Can you work these out from the model? Positions are in its coordinate system, mm. A direction names the side the tool comes from. Round coordinates to 2 decimals unless told otherwise and drop trailing zeros. Write each loop counter-clockwise with the first axis right and the second up, starting at its lowest first coordinate (ties: lowest second). Pieces come first, ordered by that corner, then holes. Notation, with made-up numbers: (13.25, -1) -> (61.25, -1) arc R26 cw to (61.25, 37) -> close; hole circle Ø11 at (27.25, 65). An arc over 180 degrees is marked (long way). Write item = value, one per line. Start each with the question number.
1) Imagine slicing it at B-B, the plane z = 10. Please give me the cut outline in (x, y).
2) Thinking about a two-plate mould opening in X: for faces 6 (the face through (-27, 17, 15)), 7 (the face through (0, 13, 17)), 8 (the face through (24.465, 23.171, 31.126)), which applies, +X half, -X half, draft (parallel to the pull), parting line (faces both ways), or undercut?
3) Imagine slicing it at A-A, the plane x = 15.5. Please give me the cut outline in (y, z).
4) Imagine slicing it at D-D, the plane x = -23. Please give me the cut outline in (y, z), then the cut area to 3 significant figures.
5) Imagine slicing it at C-C, the plane y = 22. Please give me the cut outline in (x, z).
6) If I drill on line 1 (Y direction, x = 15.5, z = 20.05); line 2 (Z direction, x = 0, y = -9.7); line 3 (X direction, y = 10.5, z = 19.65), over which ranges is the centre line in solid material (lowest first)?
7) For faces 1 (the face through (-8, -5, 0)), 2 (the face through (14, 0, 9)), 3 (the face through (0, 13, 22)), 4 (the face through (-6.5, -4, 20)), 5 (the face through (-24.535, 23.171, 31.126)), which set-ups out of +Z, -Z, +X, -X, +Y, -Y let a thin tool reach every point of the face, with its end or its side?
8) I'm going to push flat-ended pins straight in: pin 1 (10 mm diameter, centred on x = 3, y = 12.5, fed in from +Z); pin 2 (4.5 mm diameter, centred on x = -15, z = 35, fed in from +Y); pin 3 (4.5 mm diameter, centred on x = 15.5, y = 10.5, fed in from -Z); pin 4 (3 mm diameter, centred on x = 0, z = 10, fed in from -Y). Where does each tip first touch, or does it pass through?
from build123d import *

# Parameters (mm, degrees)
SKETCH113_W     = 54
SKETCH113_H     = 60
SKETCH113_R     = 11.25
SKETCH113_R_2   = 1.75
PAD070_DEPTH    = 40
SKETCH125_W     = 44
SKETCH125_H     = 50
POCKET041_DEPTH = 18.001
SKETCH126_W     = 13
SKETCH126_H     = 9
POCKET042_DEPTH = 40.001
SKETCH127_R     = 1.75
POCKET043_DEPTH = 13.001
SKETCH161_W     = 44
SKETCH161_H     = 50
POCKET060_DEPTH = 17.001
CHAMFER_SIZE2   = 47
CHAMFER_SIZE    = 18


with BuildPart() as part:
    # Sketch113 → Pad070 (new body)
    with BuildSketch(Plane.XY):
        with Locations((0, 17)):
            Rectangle(SKETCH113_W, SKETCH113_H)
        with Locations((0, 26)):
            Circle(SKETCH113_R, mode=Mode.SUBTRACT)
        with Locations((-15.5, 41.5)):
            Circle(SKETCH113_R_2, mode=Mode.SUBTRACT)
        with Locations((15.5, 41.5)):
            Circle(SKETCH113_R_2, mode=Mode.SUBTRACT)
        with Locations((15.5, 10.5)):
            Circle(SKETCH113_R_2, mode=Mode.SUBTRACT)
        with Locations((-15.5, 10.5)):
            Circle(SKETCH113_R_2, mode=Mode.SUBTRACT)
    extrude(amount=PAD070_DEPTH)

    # Sketch125 → Pocket041 (cut, through all)
    with BuildSketch(Plane.XY.offset(22)):
        with Locations((0, 25)):
            Rectangle(SKETCH125_W, SKETCH125_H)
    extrude(amount=POCKET041_DEPTH, mode=Mode.SUBTRACT)

    # Sketch126 → Pocket042 (cut, through all)
    with BuildSketch(Plane.XY):
        with Locations((0, -3.5)):
            Rectangle(SKETCH126_W, SKETCH126_H)
    extrude(amount=POCKET042_DEPTH, mode=Mode.SUBTRACT)

    # Sketch127 → Pocket043 (cut, through all)
    with BuildSketch(Plane.XZ):
        with Locations((0, 35)):
            Circle(SKETCH127_R)
        with Locations((0, 10)):
            Circle(SKETCH127_R)
    extrude(amount=POCKET043_DEPTH, mode=Mode.SUBTRACT)

    # Sketch161 → Pocket060 (cut, through all)
    with BuildSketch(Plane.XY.offset(17)):
        with Locations((0, 25)):
            Rectangle(SKETCH161_W, SKETCH161_H)
    extrude(amount=-POCKET060_DEPTH, mode=Mode.SUBTRACT)

    # Chamfer
    chamfer_edges = [part.edges().sort_by_distance(p)[0] for p in [
        (24.5, 47, 40),
        (-24.5, 47, 40),
    ]]
    chamfer_side = part.faces().sort_by_distance((0, 47, 19.822581))[0]
    chamfer(chamfer_edges, length=CHAMFER_SIZE, length2=CHAMFER_SIZE2, reference=chamfer_side)


solid = part.part
Reported:
q1.outline = (-27, -13) -> (-1.75, -13) -> (-1.75, -8) -> (-6.5, -8) -> (-6.5, 0) -> (-22, 0) -> (-22, 47) -> (-27, 47) -> close; (1.75, -13) -> (27, -13) -> (27, 47) -> (22, 47) -> (22, 0) -> (6.5, 0) -> (6.5, -8) -> (1.75, -8) -> close
q2.face_6 = -X half
q2.face_7 = undercut
q2.face_8 = draft
q3.outline = (-13, 0) -> (0, 0) -> (0, 17) -> (8.75, 17) -> (8.75, 22) -> (0, 22) -> (0, 40) -> (-13, 40) -> close; (12.25, 17) -> (39.75, 17) -> (39.75, 22) -> (12.25, 22) -> close; (43.25, 17) -> (47, 17) -> (47, 22) -> (43.25, 22) -> close
q4.outline = (-13, 0) -> (47, 0) -> (47, 22) -> (0, 40) -> (-13, 40) -> close
q4.area = 1,980 mm²
q5.outline = (-27, 0) -> (-22, 0) -> (-22, 17) -> (-10.51, 17) -> (-10.51, 22) -> (-22, 22) -> (-22, 31.57) -> (-27, 31.57) -> close; (10.51, 17) -> (22, 17) -> (22, 0) -> (27, 0) -> (27, 31.57) -> (22, 31.57) -> (22, 22) -> (10.51, 22) -> close
q6.line_1 = -13 to 8.75, 12.25 to 39.75, 43.25 to 47
q6.line_2 = 0 to 8.25, 11.75 to 33.25, 36.75 to 40
q6.line_3 = -27 to -17.25, -13.75 to 13.75, 17.25 to 27
q7.face_1 = -Z, +X, -X, +Y, -Y
q7.face_2 = -Z, +Y
q7.face_3 = +Z, +Y
q7.face_4 = +Z, -Z
q7.face_5 = +Z, +X, -X, +Y
q8.pin_1 = 22
q8.pin_2 = 0
q8.pin_3 = 17
q8.pin_4 = through
